```python
from build123d import *

# Parameters (mm, degrees)
F0_W     = 50.8
F0_H     = 25.4
F1_DEPTH = 38.1
F2_W     = 19.05
F2_H     = 12.7
F3_DEPTH = 19.05
F5_DEPTH = 12.7


with BuildPart() as f1:
    # F0 (on Front) → F1 (new body)
    with BuildSketch(Plane.XZ):
        with Locations((25.4, 12.7)):
            Rectangle(F0_W, F0_H)
    extrude(amount=F1_DEPTH)

    # F2 (on face) → F3 (cut)
    with BuildSketch(Plane.YZ.offset(50.8)):
        with Locations((-9.525, 19.05)):
            Rectangle(F2_W, F2_H)
    extrude(amount=-F3_DEPTH, mode=Mode.SUBTRACT)

    # F4 (on face) → F5 (cut)
    with BuildSketch(Plane.XY.offset(25.4)):
        Polygon((41.275, -38.1), (50.8, -19.05), (31.75, -19.05), (31.75, 0), (6.35, -38.1), align=None)
    extrude(amount=-F5_DEPTH, mode=Mode.SUBTRACT)


solid = f1.part
```
Verification items for the finished model (mm, model axes). A direction names the side the tool comes from. Coordinates: 2 decimals unless noted, no trailing zeros. Order: outer loops, then holes, each group sorted by start corner. A loop starts at its lowest first (then second) coordinate and runs counter-clockwise, first axis right, second up. Notation, with made-up numbers: (69, 27.25) -> (80, 27.25) arc R19 cw to (80, 48.25) -> close; hole circle Ø6 at (80.5, -18). An arc over 180 degrees is marked (long way). Answer as CSV lines item,"result". Start each with the question number.
1) Cross-section at D-D, the plane y = -24.5. Record the boundary of the cut face in (x, z) (3 decimals).
2) Cross-section at C-C, the plane y = -4.5. Record the boundary of the cut face in (x, z).
3) Cross-section at A-A, the plane z = 21.5. Record the boundary of the cut face in (x, y) (3 decimals).
4) Release check for a two-part mould opening along X. For faces 1 (the face through (25, -38.1, 10)), 2 (the face through (45.97, -28.71, 19.14)), 3 (the face through (0, -19, 13)) record: released by +X, released by -X, zero draft, split by the parting line, or undercut.
5) Gauge pin test, flat end, axial feed: pin 1 Ø4 at (x, z) = (10.5, 20) entering from -Y (3 decimals). Record the tip position at first contact, or that the pin passes through.
6) Cross-section at B-B, the plane x = 46.5. Record the boundary of the cut face in (y, z).
7) Set-up check for faces 4 (the face through (25, -19, 0)), 5 (the face through (34, -19, 12.7)), 6 (the face through (19.23, -18.78, 19.14)): record each of +Z, -Z, +X, -X, +Y, -Y from which the full face is reachable in a straight line by a thin tool's end or side.
8) Material ranges on L1, parallel to Z at x = 20.5, y = -28; L2, parallel to X at y = -31, z = 19.25 (3 decimals); L3, parallel to Y at x = 27.5, z = 14 (3 decimals), recorded low to high. Write a range as [from, to].
Conclusion:
1,outline,"(0, 0) -> (50.8, 0) -> (50.8, 25.4) -> (48.075, 25.4) -> (48.075, 12.7) -> (15.417, 12.7) -> (15.417, 25.4) -> (0, 25.4) -> close"
2,outline,"(0, 0) -> (50.8, 0) -> (50.8, 12.7) -> (28.75, 12.7) -> (28.75, 25.4) -> (0, 25.4) -> close"
3,outline,"(0, -38.1) -> (6.35, -38.1) -> (31.75, 0) -> (0, 0) -> close; (41.275, -38.1) -> (50.8, -38.1) -> (50.8, -19.05) -> close"
4,face 1,"zero draft"
4,face 2,"undercut"
4,face 3,"released by -X"
5,pin 1,"stops at y = -34.875"
6,outline,"(-38.1, 0) -> (0, 0) -> (0, 12.7) -> (-27.65, 12.7) -> (-27.65, 25.4) -> (-38.1, 25.4) -> close"
7,face 4,"-Z, +X, -X, +Y, -Y"
7,face 5,"+Z"
7,face 6,"+Z, -Y"
8,L1,"z = [0, 12.7]"
8,L2,"x = [0, 11.083], [44.825, 50.8]"
8,L3,"y = [-6.375, 0]"
